Geometry: see drawing. Coordinates: mm, zero at the bounding-box minimum. A direction names the side the tool comes from. Give positions to 0.01 mm unless a question says otherwise; leave off trailing zeros. Loops run counter-clockwise (first coordinate to the right, second up) from the corner with the lowest first, then second, coordinate; pieces in that order, holes last. Notation, with made-up numbers: M 85,-32 L 132,-32 A25 ccw 132,-13 Z; hole C -12,76 d4. An arc over 180 degrees is marked long. Put each result on its own line as item: value.
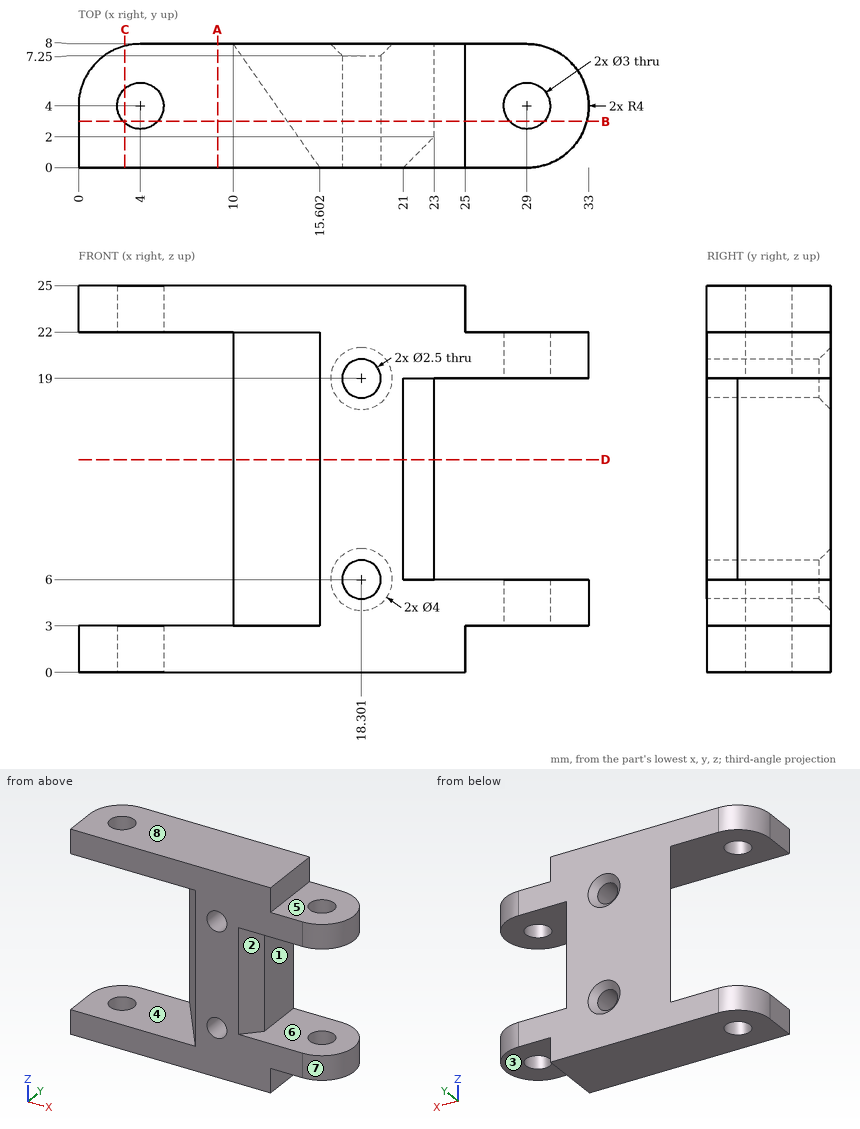
1. Draft query along Z for the marked faces 6, 7 and 8. Return one class per face: pulls with the +Z half, pulls with the -Z half, needs draft (parallel to the pull), parting line crosses it, or undercut.
Found:
face 6: undercut
face 7: needs draft
face 8: pulls with the +Z half
2. Section query D-D (z = 13.75). Output: boundary loops of the cut face in (x, y), plus the area to 3 significant figures.
Found:
outline: M 10,8 L 15.6,0 L 21,0 L 23,2 L 23,8 Z
area: 79.6 mm^2
3. Access query for the marked faces 1, 2, 3, 4 and 5. Directions: +Z, -Z, +X, -X, +Y, -Y. A direction counts if a zero-diameter tool reaches every point of the face in a straight line with its end or side. Return the directions, or none.
Found:
face 1: +X, +Y, -Y
face 2: +X, -Y
face 3: -Z, +X, +Y, -Y
face 4: -X, -Y
face 5: +Z, +X, +Y, -Y
4. Material intervals for line 1 (X direction, y = 4, z = 23); line 2 (Z direction, x = 29, y = 7.75); line 3 (Z direction, x = 4.5, y = 5.75), sorted ascending. Write a range as from..to.
Found:
line 1: 0..2.5, 5.5..25
line 2: 3..6, 19..22
line 3: 0..3, 22..25
5. Contact query for flat-ended pins moving along their axis: P1, Ø2.5, axis at y = 5, z = 1.5, coming from the +X side; P2, Ø4, axis at y = 1, z = 18, coming from the -X side; P3, Ø1.8, axis at y = 4.5, z = 15, coming from the +X side. Output: stop coordinate, or through.
Found:
P1: x = 25
P2: x = 13.5
P3: x = 23
6. Section query C-C (x = 3). Output: boundary loops of the cut face in (y, z).
Found:
outline: M 0,0 L 2.88,0 L 2.88,3 L 0,3 Z; M 0,22 L 2.88,22 L 2.88,25 L 0,25 Z; M 5.12,0 L 7.87,0 L 7.87,3 L 5.12,3 Z; M 5.12,22 L 7.87,22 L 7.87,25 L 5.12,25 Z
7. Section query A-A (x = 9). Output: boundary loops of the cut face in (y, z).
Found:
outline: M 0,0 L 8,0 L 8,3 L 0,3 Z; M 0,22 L 8,22 L 8,25 L 0,25 Z
8. Section query B-B (y = 3). State how many separate pieces and enclosed holes the cut face has, plus the area to 3 significant figures.
Found:
separate pieces: 5
enclosed holes: 2
area: 353 mm^2
